Can you work these out from the model? Positions are in its coordinate system, mm. A direction names the side the tool comes from. Round coordinates to 2 decimals unless told otherwise and drop trailing zeros. Loops run counter-clockwise (first coordinate to the right, second up) from the corner with the lowest first, then second, coordinate; pieces in that order, holes last.
from build123d import *

# Parameters (mm, degrees)
BOSS_EXTRUDE1_DEPTH = 25.4
SKETCH2_W           = 35.56
SKETCH2_H           = 32.385
CUT_EXTRUDE1_DEPTH  = 2.27838
SKETCH3_R           = 4.7879
CUT_EXTRUDE2_DEPTH  = 2.27838
SKETCH4_R           = 1.68275
CUT_EXTRUDE3_DEPTH  = 2.27838
SKETCH5_R           = 1.68275
CUT_EXTRUDE4_DEPTH  = 2.27838
CUT_EXTRUDE5_DEPTH  = 2.27838
CUT_EXTRUDE6_DEPTH  = 2.27838


with BuildPart() as part:
    # Sketch1 → Boss-Extrude1 (new body)
    with BuildSketch(Plane(origin=(0, 0, 0), x_dir=(0, 0, -1), z_dir=(1, 0, 0))):
        with BuildLine():
            Line((-9.525, 1.51892), (-9.525, 0))
            Line((-9.525, 0), (-2.28092, 0))
            ThreePointArc((-2.28092, 0), (-0.668066001, 0.668066001), (0, 2.28092))
            Line((0, 2.28092), (0, 22.86))
            Line((0, 22.86), (-1.51892, 22.86))
            Line((-1.51892, 22.86), (-1.51892, 2.28092))
            ThreePointArc((-1.51892, 2.28092), (-1.742104633, 1.742104633), (-2.28092, 1.51892))
            Line((-2.28092, 1.51892), (-9.525, 1.51892))
        make_face()
    extrude(amount=BOSS_EXTRUDE1_DEPTH)

    # Sketch2 → Cut-Extrude1 (cut)
    with BuildSketch(Plane.XY):
        with Locations((12.7, 14.2875)):
            Rectangle(SKETCH2_W, SKETCH2_H)
        with BuildLine():
            Line((-1.550018352, 0), (26.950018352, 0))
            Line((26.950018352, 0), (19.821465766, 14.601862247))
            ThreePointArc((19.821465766, 14.601862247), (12.7, 19.05), (5.578534234, 14.601862247))
            Line((5.578534234, 14.601862247), (-1.550018352, 0))
        make_face(mode=Mode.SUBTRACT)
    extrude(amount=CUT_EXTRUDE1_DEPTH, mode=Mode.SUBTRACT)

    # Sketch3 → Cut-Extrude2 (cut)
    with BuildSketch(Plane.XY):
        with Locations((12.7, 11.1252)):
            Circle(SKETCH3_R)
    extrude(amount=CUT_EXTRUDE2_DEPTH, mode=Mode.SUBTRACT)

    # Sketch4 → Cut-Extrude3 (cut)
    with BuildSketch(Plane(origin=(0, 0, 0), x_dir=(1, 0, 0), z_dir=(0, 1, 0))):
        with Locations((3.175, -6.35)):
            Circle(SKETCH4_R)
    extrude(amount=CUT_EXTRUDE3_DEPTH, mode=Mode.SUBTRACT)

    # Sketch5 → Cut-Extrude4 (cut)
    with BuildSketch(Plane(origin=(0, 0, 0), x_dir=(1, 0, 0), z_dir=(0, 1, 0))):
        with Locations((22.225, -6.35)):
            Circle(SKETCH5_R)
    extrude(amount=CUT_EXTRUDE4_DEPTH, mode=Mode.SUBTRACT)

    # Sketch6 → Cut-Extrude5 (cut)
    with BuildSketch(Plane(origin=(0, 0, 0), x_dir=(1, 0, 0), z_dir=(0, 1, 0))):
        with BuildLine():
            Line((-12.7, -12.7), (3.175, -12.7))
            Line((3.175, -12.7), (3.175, -9.525))
            ThreePointArc((3.175, -9.525), (0.92993597, -8.59506403), (0, -6.35))
            Line((0, -6.35), (-12.7, -6.35))
            Line((-12.7, -6.35), (-12.7, -12.7))
        make_face()
    extrude(amount=CUT_EXTRUDE5_DEPTH, mode=Mode.SUBTRACT)

    # Sketch7 → Cut-Extrude6 (cut)
    with BuildSketch(Plane(origin=(0, 0, 0), x_dir=(1, 0, 0), z_dir=(0, 1, 0))):
        with BuildLine():
            Line((22.225, -9.525), (22.225, -12.7))
            Line((22.225, -12.7), (38.1, -12.7))
            Line((38.1, -12.7), (38.1, -6.35))
            Line((38.1, -6.35), (25.4, -6.35))
            ThreePointArc((25.4, -6.35), (24.47006403, -8.59506403), (22.225, -9.525))
        make_face()
    extrude(amount=CUT_EXTRUDE6_DEPTH, mode=Mode.SUBTRACT)


solid = part.part
(1) If we section it at A-A, the plane x = 12.7: List the corners of the cut face in (y, z) for me (3 decimals).
Worked answers:
outline: (0, 2.281) arc R2.281 ccw to (2.281, 0) - (6.337, 0) - (6.337, 1.519) - (2.281, 1.519) arc R0.762 cw to (1.519, 2.281) - (1.519, 9.525) - (0, 9.525) - close; (15.913, 0) - (19.05, 0) - (19.05, 1.519) - (15.913, 1.519) - close
(2) If we section it at D-D, the plane x = 6.5: List the corners of the cut face in (y, z) for me (3 decimals).
Worked answers:
outline: (0, 2.281) arc R2.281 ccw to (2.281, 0) - (16.061, 0) - (16.061, 1.519) - (2.281, 1.519) arc R0.762 cw to (1.519, 2.281) - (1.519, 9.525) - (0, 9.525) - close
(3) Will these pins go through, and if not, where does the flat tip stop? P1, Ø3, axis at x = 3, y = 14.5, coming from the +Z side; P2, Ø8.5, axis at x = 10.5, y = 12.5, coming from the +Z side; P3, Ø3, axis at x = 8.5, z = 8, coming from the +Y side; P4, Ø2, axis at x = 4.5, z = 3, coming from the +Y side.
Worked answers:
P1: passes through
P2: stops at z = 1.52
P3: stops at y = 1.52
P4: stops at y = 1.57
(4) If we section it at B-B, the plane y = 13.25: List the corners of the cut face in (x, z) for me.
Worked answers:
outline: (4.92, 0) - (8.41, 0) - (8.41, 1.52) - (4.92, 1.52) - close; (16.99, 0) - (20.48, 0) - (20.48, 1.52) - (16.99, 1.52) - close
(5) If I drill on line 1 (X direction, y = 0.3, z = 6.35); line 2 (Y direction, x = 13.5, z = 2.5), over which ranges is the centre line in solid material (lowest first)?
Worked answers:
line 1: x = 0 to 1.49, 4.86 to 20.54, 23.91 to 25.4
line 2: y = 0 to 1.52
(6) For faces 4 (the flat face through (22.65, 8.81, 0.75)), 5 (the flat face through (9.7, 7.1, 1.519)), which set-ups out of +Z, -Z, +X, -X, +Y, -Y let a thin tool reach every point of the face, with its end or its side?
Worked answers:
face 4: +Z, -Z, +X, +Y
face 5: +Z, +X, -X, +Y
(7) If we mould it in two halves opening along Y, with no side actions, what happens to faces 1 (the flat face through (13, 0, 6)), 2 (the cylindrical face through (7.917, 11.336, 0.749)), 3 (the cylindrical face through (23.83, 0.75, 5.84))? For each: released by +Y, released by -Y, zero draft, split by the parting line, or undercut.
Worked answers:
face 1: released by -Y
face 2: undercut
face 3: zero draft
(8) If we section it at C-C, the plane z = 1: List the corners of the cut face in (x, y) for me (3 decimals).
Worked answers:
outline: (0, 0.394) - (25.4, 0.394) - (25.4, 3.175) - (19.821, 14.602) arc R7.925 ccw to (5.579, 14.602) - (0, 3.175) - close; hole circle Ø9.576 at (12.7, 11.125)
